Design review of the part built by this model. Coordinates are the model's own, in mm. Coordinates: 2 decimals unless noted, no trailing zeros. Loops run counter-clockwise (first coordinate to the right, second up) from the corner with the lowest first, then second, coordinate; pieces in that order, holes last. Notation, with made-up numbers: (41.25, 18) - (52.25, 18) arc R27 ccw to (52.25, 35) - close; hole circle Ø8 at (-31, 15.5). An arc over 180 degrees is marked (long way). Use one line per item in the form item = value. Start each with the question number.
(1) Clearance check with flat-ended pins moving along their axes: pin 1 Ø1.5 at (x, z) = (14.5, 1) entering from +Y; pin 2 Ø1.5 at (y, z) = (-77, 2) entering from -X; pin 3 Ø1.5 at (x, z) = (77, 2) entering from +Y. State where each tip first meets the part, or that it passes through.
(2) Add section A-A (x = 12.5). State the section outline as (y, z) points, plus the area to 3 significant figures.
(3) For L1, parallel to X at y = -21, z = 0.25, list the stretches that pass through material, from the lowest coordinate up.
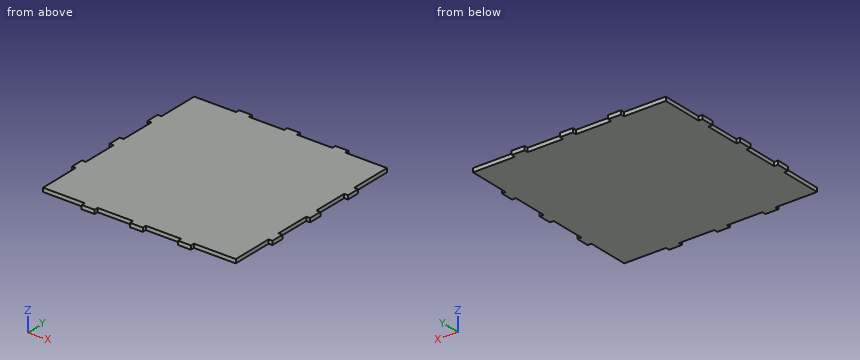
Autodesk Inventor part; units mm, degrees
ref_plane "YZ Plane" through (0, 0, 0) normal (1, 0, 0) x (0, 1, 0)
ref_plane "XZ Plane" through (0, 0, 0) normal (0, 1, 0) x (-1, 0, 0)
ref_plane "XY Plane" through (0, 0, 0) normal (0, 0, 1) x (1, 0, 0)
sketch "Эскиз1" plane through (0, 0, 0) normal (0, 0, 1) x (1, 0, 0)
  line L0 (-78, 42.5) -> (-75, 42.5)
  line L1 (-75, 32.5) -> (-78, 32.5)
  line L2 (-78, 32.5) -> (-78, 42.5)
  line L3 (-78, 5) -> (-75, 5)
  line L4 (-78, 0) -> (-78, 5)
  line L5 (-42.5, 78) -> (-32.5, 78)
  line L6 (-32.5, 78) -> (-32.5, 75)
  line L7 (-42.5, 75) -> (-42.5, 78)
  line L8 (-5, 78) -> (0, 78)
  line L9 (-5, 75) -> (-5, 78)
  line L10 (-5, 75) -> (-32.5, 75)
  line L11 (-42.5, 75) -> (-75, 75)
  line L12 (-75, 75) -> (-75, 42.5)
  line L13 (-75, 32.5) -> (-75, 5)
  line L14 (75, 32.5) -> (78, 32.5)
  line L15 (75, 5) -> (75, 32.5)
  line L16 (78, 5) -> (75, 5)
  line L17 (78, 0) -> (78, 5)
  line L18 (78, 42.5) -> (75, 42.5)
  line L19 (78, 32.5) -> (78, 42.5)
  line L20 (5, 75) -> (32.5, 75)
  line L21 (5, 78) -> (0, 78)
  line L22 (5, 75) -> (5, 78)
  line L23 (75, 75) -> (75, 42.5)
  line L24 (42.5, 75) -> (75, 75)
  line L25 (32.5, 78) -> (32.5, 75)
  line L26 (42.5, 78) -> (32.5, 78)
  line L27 (42.5, 75) -> (42.5, 78)
  line L28 (32.5, -78) -> (32.5, -75)
  line L29 (5, -75) -> (32.5, -75)
  line L30 (5, -75) -> (5, -78)
  line L31 (5, -78) -> (0, -78)
  line L32 (-5, -78) -> (0, -78)
  line L33 (-5, -75) -> (-5, -78)
  line L34 (-5, -75) -> (-32.5, -75)
  line L35 (-32.5, -78) -> (-32.5, -75)
  line L36 (-78, -42.5) -> (-75, -42.5)
  line L37 (-78, -32.5) -> (-78, -42.5)
  line L38 (-42.5, -78) -> (-32.5, -78)
  line L39 (-42.5, -75) -> (-75, -75)
  line L40 (-42.5, -75) -> (-42.5, -78)
  line L41 (-75, -75) -> (-75, -42.5)
  line L42 (-75, -32.5) -> (-78, -32.5)
  line L43 (-78, -5) -> (-75, -5)
  line L44 (-78, 0) -> (-78, -5)
  line L45 (-75, -5) -> (-75, -32.5)
  line L46 (75, -32.5) -> (78, -32.5)
  line L47 (78, -42.5) -> (75, -42.5)
  line L48 (78, -32.5) -> (78, -42.5)
  line L49 (75, -32.5) -> (75, -5)
  line L50 (78, -5) -> (75, -5)
  line L51 (78, 0) -> (78, -5)
  line L52 (42.5, -78) -> (32.5, -78)
  line L53 (42.5, -75) -> (42.5, -78)
  line L54 (42.5, -75) -> (75, -75)
  line L55 (75, -42.5) -> (75, -75)
  point P0 (0, 0)
  point P1 (0, 0)
  point P2 (0, 0)
extrude "Выдавливание1" add sketch "Эскиз1" along normal blind 3
properties part number "Низ"
Computed values:
q1.pin_1 = 75
q1.pin_2 = -42.5
q1.pin_3 = 42.5
q2.outline = (-75, 0) - (75, 0) - (75, 3) - (-75, 3) - close
q2.area = 450 mm^2
q3.L1 = -75 to 75
